from build123d import *

# Parameters (mm, degrees)
SKETCH1_R           = 0.405
SKETCH1_R_2         = 0.255
BOSS_EXTRUDE1_DEPTH = 150
CUT_EXTRUDE1_DEPTH  = 0.5


with BuildPart() as part:
    # Sketch1 → Boss-Extrude1 (new body)
    with BuildSketch(Plane.XY):
        Circle(SKETCH1_R)
        Circle(SKETCH1_R_2, mode=Mode.SUBTRACT)
    extrude(amount=BOSS_EXTRUDE1_DEPTH)

    # Sketch2 → Cut-Extrude1 (cut, symmetric)
    with BuildSketch(Plane(origin=(0, 0, 0), x_dir=(0, 0, -1), z_dir=(1, 0, 0))):
        Polygon((-150, -0.405), (-148.514947888, 0.195), (-148.514947888, -0.055), (-146.014947888, -0.055), (-146.014947888, 0.595), (-150.3, 0.595), (-150.3, -0.405), align=None)
    extrude(amount=CUT_EXTRUDE1_DEPTH, both=True, mode=Mode.SUBTRACT)


solid = part.part
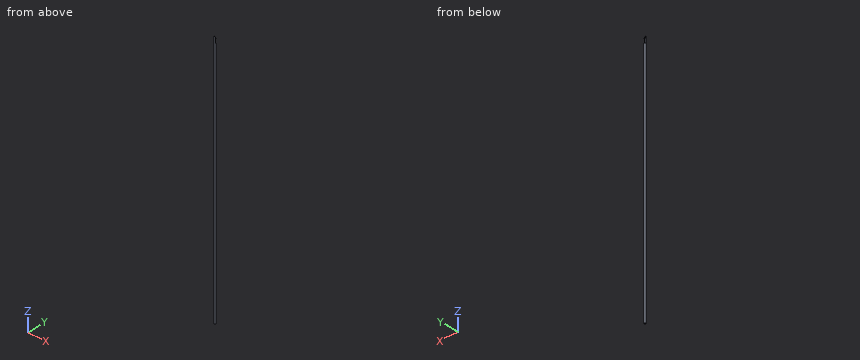
The listing builds one solid part. Answer for the finished solid, in the listing's coordinates (mm). Give positions to 0.01 mm unless a question says otherwise; leave off trailing zeros. Write each loop counter-clockwise with the first axis right and the second up, starting at its lowest first coordinate (ties: lowest second). Pieces come first, ordered by that corner, then holes.
Item 1: Section B-B, the plane z = 118.5 is taken. Write down the section's boundary in (x, y) (3 decimals).
Item 2: Find the intervals of material crossed by line 1 along Y through (x, z) = (0.1, 63); line 2 along Y through (x, z) = (0.05, 67.5), in increasing order.
Item 3: Section A-A, the plane x = 0 is taken. Write down the section's boundary in (y, z) (3 decimals).
Completed:
1. outline: circle Ø0.81 at (0, 0); hole circle Ø0.51 at (0, 0)
2. line 1: y = -0.39 to -0.23, 0.23 to 0.39
2. line 2: y = -0.4 to -0.25, 0.25 to 0.4
3. outline: (-0.405, 0) - (-0.255, 0) - (-0.255, 149.629) - (-0.405, 150) - close; (0.255, 0) - (0.405, 0) - (0.405, 146.015) - (0.255, 146.015) - close
